Autodesk Inventor part; units mm, degrees
ref_plane "YZ Plane" through (0, 0, 0) normal (1, 0, 0) x (0, 1, 0)
ref_plane "XZ Plane" through (0, 0, 0) normal (0, 1, 0) x (-1, 0, 0)
ref_plane "XY Plane" through (0, 0, 0) normal (0, 0, 1) x (1, 0, 0)
sketch "Sketch1" plane through (0, 0, 0) normal (0, 0, 1) x (1, 0, 0)
  line L0 (-22.325, 20) -> (-22.325, 0)
  line L1 (-22.325, 0) -> (-23.9, 0)
  line L2 (-23.9, 0) -> (-23.9, 6)
  line L3 (-23.9, 6) -> (-25.325, 6)
  line L4 (-25.325, 6) -> (-25.325, 16)
  line L5 (-25.325, 16) -> (-30, 16)
  line L6 (-30, 16) -> (-30, 28)
  line L7 (-30, 28) -> (-26.5, 28)
  line L8 (-26.5, 28) -> (-26.5, 20)
  line L9 (-26.5, 20) -> (-22.325, 20)
  line L10 (0, -5.6) -> (0, 33.6)
  point P0 (0, 0)
  dimension "d0" = 23.9
  dimension "neck_ir" = 22.325
  dimension "d4" = 8
  dimension "d5" = 6
  dimension "d6" = 3
  dimension "d7" = 10
  dimension "neck_thread_dia" = 30
  dimension "neck_thread_len" = 12
  dimension "d14" = 26.5
revolve "Revolution1" add sketch "Sketch1" angle 360 about axis through (0, -10, 0) along (0, 1, 0)
thread "Thread1"
equation "\"d4\" = 2 * oring_dia"
equation "\"d14\" = 0.5 * oring_od"
equation "\"oring_diameter\" = 4"
properties part number "neck" material "Brass"
Can you work these out from the model? Positions are in its coordinate system, mm. A direction names the side the tool comes from. Round coordinates to 2 decimals unless told otherwise and drop trailing zeros. Loops run counter-clockwise (first coordinate to the right, second up) from the corner with the lowest first, then second, coordinate; pieces in that order, holes last. Notation, with made-up numbers: (-26, -7) -> (-7, -7) arc R31 ccw to (-7, 29) -> close; hole circle Ø7 at (-4.75, -19). An arc over 180 degrees is marked (long way). One line per item, written item: value. Start each with the question number.
1. For pin 1 (6 mm diameter, centred on x = 4, y = 14.5, fed in from -Z); pin 2 (2 mm diameter, centred on x = -17, y = 23, fed in from +Z); pin 3 (8 mm diameter, centred on y = 21.5, z = -18, fed in from -X), each with a flat end and sliding along its axis, tell me the tip position at first contact or that it passes through.
2. If we section it at B-B, the plane x = 0: Write out the boundary of the cut face in (y, z) (3 decimals).
3. For faces 1 (the cylindrical face through (-14.246, 23.944, -22.345)), 2 (the cylindrical face through (29.97, 22.08, 1.32)), 3 (the cylindrical face through (-12.85, 3.04, 20.15)), which set-ups out of +Z, -Z, +X, -X, +Y, -Y let a thin tool reach every point of the face, with its end or its side?
4. If I drill on probe 1 along X at (y, z) = (22.75, -0.5); probe 2 along Z at (x, y) = (0.5, 11), over which ranges is the centre line in solid material (lowest first)?
5. If we section it at D-D, the plane y = 18.25: Write out the boundary of the cut face in (x, z) (3 decimals).
6. If we mould it in two halves opening along X, with no side actions, what happens to faces 4 (the cylindrical face through (4.84, 9.86, 21.794)), 5 (the flat face through (25, 16, -7)), 6 (the cylindrical face through (5.49, 11.07, -24.723)), 7 (the flat face through (14, 20, -18))? For each: pulls with the +X half, pulls with the -X half, needs draft (parallel to the pull), parting line crosses it, or undercut.
7. If we section it at C-C, the plane y = 3.75: Write out the boundary of the cut face in (x, z) (3 decimals), then the cut area to 3 significant figures.
8. If we section it at A-A, the plane z = 0: Write out the boundary of the cut face in (x, y) (3 decimals), then the cut area to 3 significant figures.
Calculated:
1. pin 1: stops at z = -29.97
1. pin 2: stops at z = 25.38
1. pin 3: stops at x = -26.53
2. outline: (0, -23.9) -> (6, -23.9) -> (6, -25.325) -> (16, -25.325) -> (16, -30) -> (28, -30) -> (28, -26.5) -> (20, -26.5) -> (20, -22.325) -> (0, -22.325) -> close; (0, 22.325) -> (20, 22.325) -> (20, 26.5) -> (28, 26.5) -> (28, 30) -> (16, 30) -> (16, 25.325) -> (6, 25.325) -> (6, 23.9) -> (0, 23.9) -> close
3. face 1: +Y
3. face 2: +Y, -Y
3. face 3: -Y
4. probe 1: x = -30 to -26.5, 26.5 to 30
4. probe 2: z = -25.32 to -22.32, 22.32 to 25.32
5. outline: circle Ø60 at (0, 0); hole circle Ø44.65 at (0, 0)
6. face 4: undercut
6. face 5: needs draft
6. face 6: parting line crosses it
6. face 7: undercut
7. outline: circle Ø47.8 at (0, 0); hole circle Ø44.65 at (0, 0)
7. area: 229 mm²
8. outline: (-30, 16) -> (-25.325, 16) -> (-25.325, 6) -> (-23.9, 6) -> (-23.9, 0) -> (-22.325, 0) -> (-22.325, 20) -> (-26.5, 20) -> (-26.5, 28) -> (-30, 28) -> close; (22.325, 0) -> (23.9, 0) -> (23.9, 6) -> (25.325, 6) -> (25.325, 16) -> (30, 16) -> (30, 28) -> (26.5, 28) -> (26.5, 20) -> (22.325, 20) -> close
8. area: 196 mm²
